Solid Edge part; units mm, degrees
sketch "Sketch1" plane through (0, 0, 0) normal (0, 0, 1) x (1, 0, 0)
  circle A0 centre (-37.5833, 45.3496) radius 200
extrude "Protrusion1" add sketch "Sketch1" along normal blind 630
sketch "Sketch2" plane through (-37.5833, 45.3496, -30) normal (0, 0, -1) x (0, -1, 0)
  circle A0 centre (0, 0) radius 25
extrude "Cutout1" cut sketch "Sketch2" against normal through all
sketch "Sketch3" plane through (-37.5833, 45.3496, 630) normal (0, 0, 1) x (0, 1, 0)
  circle A0 centre (0, 0) radius 185
extrude "Cutout2" cut sketch "Sketch3" against normal through all
sketch "Sketch4" plane through (-37.5833, 45.3496, 0) normal (0, 0, -1) x (0, 1, 0)
  circle A0 centre (0, 192.5) radius 5
extrude "ExtrudedCutout_4" cut sketch "Sketch4" against normal blind 10
pattern_circular "Pattern1" count 10 over 360 about axis through (-37.5833, 45.3496, 0) along (0, 0, 1) of "ExtrudedCutout_4"
mirror "Mirror1" about plane through (-37.5833, 45.3496, 315) normal (0, 0, 1) of "ExtrudedCutout_4", "Pattern1"
properties material "Aluminum, 6061-T6"
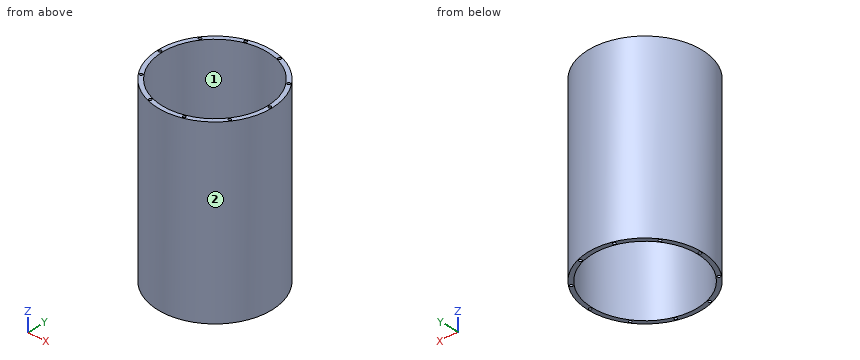
Geometry check sheet. Reference: the model listing, model coordinates, mm. Face numbers are marked on the shaded views. Coordinates: 2 decimals unless noted, no trailing zeros. Order: outer loops, then holes, each group sorted by start corner. A loop starts at its lowest first (then second) coordinate and runs counter-clockwise, first axis right, second up. Notation, with made-up numbers: (31, 73.25) - (68, 73.25) arc R19 ccw to (68, 79.25) - close; hole circle Ø9 at (40, 50.5). An arc over 180 degrees is marked (long way). One line per item, written item: value.
(1) Thickness scan on probe 1 along Y at (x, z) = (-37, 247); probe 2 along X at (y, z) = (162, 318.5); probe 3 along Y at (x, z) = (107, 92). Record the ranges inside material, lowest first. Write a range as from..to.
Data:
probe 1: y = -154.65..-139.65, 230.35..245.35
probe 2: x = -200.04..-181.17, 106.01..124.87
probe 3: y = -92.84..-70.07, 160.76..183.54
(2) Sectioned sample at B-B (x = -17.5). Enter the section's corners in (y, z), and give its area (3 significant figures).
Data:
outline: (-153.64, 0) - (-138.56, 0) - (-138.56, 630) - (-153.64, 630) - close; (229.26, 0) - (244.34, 0) - (244.34, 630) - (229.26, 630) - close
area: 19,000 mm^2
(3) Depth check by flat-ended pin: pin 1 Ø6 at (x, z) = (-118, 82) entering from -Y; pin 2 Ø16 at (x, y) = (118.15, 158.5) entering from -Z; pin 3 Ø3 at (x, z) = (-54.5, 520.5) entering from +Y; pin 4 Ø3 at (x, y) = (154, 44.5) entering from +Z. Enter the tip coordinate at first touch or a pass-through.
Data:
pin 1: stops at y = -139.06
pin 2: stops at z = 0
pin 3: stops at y = 244.75
pin 4: stops at z = 620
(4) Release check for a two-part mould opening along X. For the marked faces 1 and 2 record: +X half, -X half, draft (parallel to the pull), parting line (faces both ways), or undercut.
Data:
face 1: undercut
face 2: parting line
(5) Sectioned sample at A-A (y = -32). Enter the section's corners in (x, z), and give its area (3 significant figures).
Data:
outline: (-222.02, 0) - (-205.64, 0) - (-205.64, 630) - (-222.02, 630) - close; (130.47, 0) - (146.85, 0) - (146.85, 630) - (130.47, 630) - close
area: 20,600 mm^2
(6) Sectioned sample at C-C (z = 334). Enter the section's corners in (x, y).
Data:
outline: circle Ø400 at (-37.58, 45.35); hole circle Ø370 at (-37.58, 45.35)
